The figure shows three views and two pictorial views of one solid part (mm, origin at its lowest corner). Answer the questions. A direction names the side the tool comes from. Coordinates: 2 decimals unless noted, no trailing zeros. Order: outer loops, then holes, each group sorted by start corner. A loop starts at its lowest first (then second) coordinate and runs counter-clockwise, first axis right, second up. Notation, with made-up numbers: (-35, -4.5) -> (20, -4.5) arc R24 cw to (20, 30.5) -> close; hole circle Ø5 at (-3.75, 61.5). An arc over 180 degrees is marked (long way). Return JSON: item names as keys, results as strings. Group by question number.
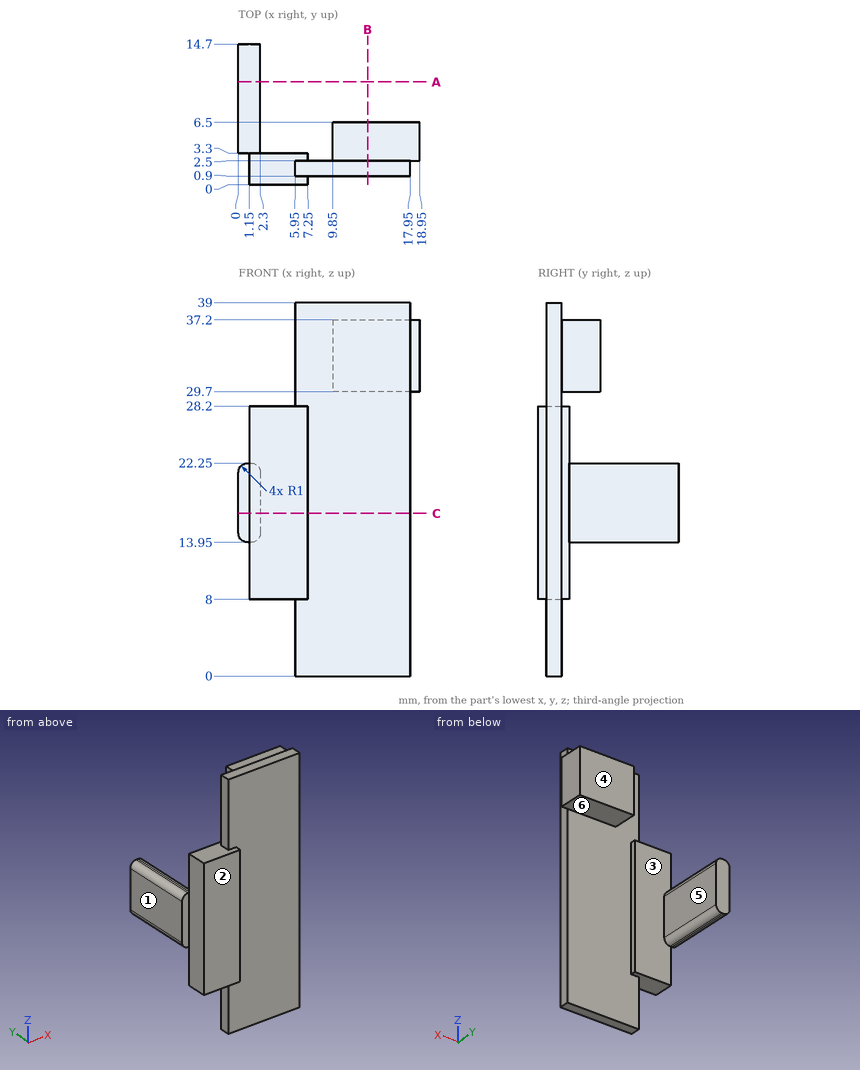
1. For a pull along Y with two mould halves and no side action, classify the marked faces 1, 2 and 3 as released by +Y, released by -Y, zero draft, split by the parting line, or undercut.
2. Straight lines are drawn through the part: L1, parallel to Y at x = 7.75, z = 2; L2, parallel to X at y = 13.75, z = 20; L3, parallel to Y at x = 5.75, z = 19.5. For each, find the intervals that lie inside material, in ascending order.
3. Given pin 1 (1.3 mm diameter, centred on y = 1.5, z = 19.5, fed in from +X); pin 2 (3.5 mm diameter, centred on x = 12, z = 11, fed in from -Y); pin 3 (0.8 mm diameter, centred on y = 2, z = 33.5, fed in from -X); pin 4 (1 mm diameter, centred on x = 5, y = 4.5, fed in from -Z), each flat-ended and moving along its own axis, determine where each tip first touches the part or whether it passes through.
4. Which of the six approach directions +Z, -Z, +X, -X, +Y, -Y give full straight-line access (tool end or side, diameter ignored) to the marked faces 4, 5 and 6?
5. Find section A-A on y = 10.75. Determine the outline of the cut face in (x, z), and give its area (3 significant figures).
6. Find section C-C on z = 17. Determine the outline of the cut face in (x, y).
7. Find section B-B on x = 13.5. Determine the outline of the cut face in (y, z).
Result:
{
 "1": {"face 1": "zero draft", "face 2": "released by -Y", "face 3": "released by +Y"},
 "2": {"L1": "0.9 to 2.5", "L2": "0 to 2.3", "L3": "0 to 3.3"},
 "3": {"pin 1": "x = 17.95", "pin 2": "y = 0.9", "pin 3": "x = 5.95", "pin 4": "through"},
 "4": {"face 4": "+Z, -Z, +X, -X, +Y", "face 5": "+Z, -Z, +X, +Y", "face 6": "-Z, +X, -X, +Y"},
 "5": {"outline": "(0, 14.95) arc R1 ccw to (1, 13.95) -> (1.3, 13.95) arc R1 ccw to (2.3, 14.95) -> (2.3, 21.25) arc R1 ccw to (1.3, 22.25) -> (1, 22.25) arc R1 ccw to (0, 21.25) -> close", "area": "18.2 mm^2"},
 "6": {"outline": "(0, 3.3) -> (1.15, 3.3) -> (1.15, 0) -> (7.25, 0) -> (7.25, 0.9) -> (17.95, 0.9) -> (17.95, 2.5) -> (7.25, 2.5) -> (7.25, 3.3) -> (2.3, 3.3) -> (2.3, 14.7) -> (0, 14.7) -> close"},
 "7": {"outline": "(0.9, 0) -> (2.5, 0) -> (2.5, 29.7) -> (6.5, 29.7) -> (6.5, 37.2) -> (2.5, 37.2) -> (2.5, 39) -> (0.9, 39) -> close"}
}
